```python
from build123d import *

# Parameters (mm, degrees)
F0_W          = 1346.2
F0_H          = 685.8
F1_DEPTH      = 25.4
F2_W          = 50.8
F2_H          = 76.2
F3_DEPTH      = 685.8
F4_W          = 1344.644603
F4_H          = 317.5
F5_DEPTH      = 38.1
F6_W          = 50.8
F6_H          = 25.4
F8_DEPTH      = 76.2
F8_DEPTH_BACK = 431.8
F7_W          = 50.8
F7_H          = 25.4
F9_DEPTH      = 76.2
F9_DEPTH_BACK = 431.8
F10_W         = 1244.6
F10_H         = 304.8
F11_DEPTH     = 25.4


with BuildPart() as f1:
    # F0 (on Top) → F1 (new body)
    with BuildSketch(Plane.XY):
        with Locations((2.175501, 32.721092)):
            Rectangle(F0_W, F0_H)
    extrude(amount=F1_DEPTH)



with BuildPart() as f3:
    # F2 (on Top) → F3 (new body)
    with BuildSketch(Plane.XY):
        with Locations((-643.969102, 185.121092)):
            Rectangle(F2_W, F2_H)
        with Locations((648.571236, 185.121092)):
            Rectangle(F2_W, F2_H)
    extrude(amount=-F3_DEPTH)


with BuildPart() as f1_1:
    add(f1.part)

    add(f3.part)  # F5 merges F3
    # F4 (on face) → F5 (join)
    with BuildSketch(Plane(origin=(0, 0, 0), x_dir=(1, 0, 0), z_dir=(0, 0, -1))):
        with Locations((2.953199, 11.728908)):
            Rectangle(F4_W, F4_H)
    extrude(amount=F5_DEPTH)

    # F6 (on face) → F8 (join, two sides)
    with BuildSketch(Plane(origin=(0, 223.221092, 0), x_dir=(-1, 0, 0), z_dir=(0, 1, 0))) as f8_sk:
        with Locations((-648.571236, -698.5)):
            Rectangle(F6_W, F6_H)
    extrude(amount=F8_DEPTH)
    extrude(f8_sk.sketch, amount=-F8_DEPTH_BACK)

    # F7 (on face) → F9 (join, two sides)
    with BuildSketch(Plane(origin=(0, 223.221092, 0), x_dir=(-1, 0, 0), z_dir=(0, 1, 0))) as f9_sk:
        with Locations((643.969102, -698.5)):
            Rectangle(F7_W, F7_H)
    extrude(amount=F9_DEPTH)
    extrude(f9_sk.sketch, amount=-F9_DEPTH_BACK)

    # F10 (on face) → F11 (join)
    with BuildSketch(Plane(origin=(0, 223.221092, 0), x_dir=(-1, 0, 0), z_dir=(0, 1, 0))):
        with Locations((-0.871236, -152.4)):
            Rectangle(F10_W, F10_H)
    extrude(amount=-F11_DEPTH)


solid = f1_1.part
```
Read the model definition and answer for the solid it produces. Units are mm, in the model's axes. A direction names the side the tool comes from. Give positions to 0.01 mm unless a question says otherwise; leave off trailing zeros. Order: outer loops, then holes, each group sorted by start corner. A loop starts at its lowest first (then second) coordinate and runs counter-clockwise, first axis right, second up.
(1) Find section D-D (x = 340). Give the vertices of the cut face in (y, z).
(2) Given pin 1 (11.5 mm diameter, centred on x = 233.5, z = -20.5, fed in from -Y); pin 2 (19 mm diameter, centred on y = -50, z = -21.5, fed in from -X); pin 3 (6 mm diameter, centred on x = -285, z = -113, fed in from -Y), each flat-ended and moving along its own axis, determine where each tip first touches the part or whether it passes through.
(3) For a pull along Y with two mould halves and no side action, classify faces 5 (the flat face through (649, 299.421, -698)), 6 (the flat face through (-644, 49, -711.2)), 7 (the flat face through (-6, 173, 0)) as released by +Y, released by -Y, zero draft, split by the parting line, or undercut.
(4) Find section B-B (y = 27). Give the vertices of the cut face in (x, z), plus the area to 3 significant figures.
(5) For faces 1 (the flat face through (-7, 38, 25.4)), 2 (the flat face through (649, 261, -685.8)), 3 (the flat face through (-669.369, 159, -410)), 4 (the flat face through (-644, 147.021, -357)), determine the directions among +Z, -Z, +X, -X, +Y, -Y from which every point of the face is accessible in a straight line to the end or side of a thin tool.
(6) Find section C-C (z = -105.5). Give the vertices of the cut face in (x, y).
(7) Find section A-A (z = -464). Give the vertices of the cut face in (x, y), plus the area to 3 significant figures.
(8) Straight lines are drawn through the part: L1, parallel to Z at x = 506.5, y = -49.5; L2, parallel to Z at x = -491, y = -213; L3, parallel to Y at x = 265, z = -74. For each, find the intervals that lie inside material, in ascending order.
Result sheet:
1. outline: (-310.18, 0) - (-170.48, 0) - (-170.48, -38.1) - (147.02, -38.1) - (147.02, 0) - (197.82, 0) - (197.82, -304.8) - (223.22, -304.8) - (223.22, 0) - (375.62, 0) - (375.62, 25.4) - (-310.18, 25.4) - close
2. pin 1: stops at y = -170.48
2. pin 2: stops at x = -669.37
2. pin 3: stops at y = 197.82
3. face 5: released by +Y
3. face 6: zero draft
3. face 7: undercut
4. outline: (-670.92, 0) - (-669.37, 0) - (-669.37, -38.1) - (675.28, -38.1) - (675.28, 25.4) - (-670.92, 25.4) - close; (-669.37, -711.2) - (-618.57, -711.2) - (-618.57, -685.8) - (-669.37, -685.8) - close; (623.17, -711.2) - (673.97, -711.2) - (673.97, -685.8) - (623.17, -685.8) - close
4. area: 88,000 mm2
5. face 1: +Z, +X, -X, +Y, -Y
5. face 2: +X, -X, +Y
5. face 3: -Z, -X, +Y, -Y
5. face 4: +X, -X, -Y
6. outline: (-669.37, 147.02) - (-618.57, 147.02) - (-618.57, 197.82) - (623.17, 197.82) - (623.17, 147.02) - (673.97, 147.02) - (673.97, 223.22) - (-669.37, 223.22) - close
7. outline: (-669.37, 147.02) - (-618.57, 147.02) - (-618.57, 223.22) - (-669.37, 223.22) - close; (623.17, 147.02) - (673.97, 147.02) - (673.97, 223.22) - (623.17, 223.22) - close
7. area: 7,740 mm2
8. L1: z = -38.1 to 25.4
8. L2: z = 0 to 25.4
8. L3: y = 197.82 to 223.22
